For this review, take the finished solid that the model builds, in its own axes (mm). Face numbers are marked on the shaded views. A direction names the side the tool comes from. Give positions to 0.01 mm unless a question says otherwise; leave off trailing zeros. Write each loop counter-clockwise with the first axis right and the second up, starting at its lowest first coordinate (ties: lowest second). Pieces come first, ordered by that corner, then holes.
Q1. For line 1 (Y direction, x = -4.75, z = 0.95); line 2 (X direction, y = 3.25, z = 2); line 3 (X direction, y = 1.25, z = -14.5), list the stretches that pass through material, from the lowest coordinate up.
Q2. We need section C-C (x = 10). Write out the cut boundary in (y, z).
Q3. We need section D-D (y = 9.8). Write out the cut boundary in (x, z), then the cut area to 3 significant figures.
Q4. We need section A-A (x = -4.75). Write out the cut boundary in (y, z), then the cut area to 3 significant figures.
Q5. Insertion check: P1, Ø5.5, axis at x = -4.75, y = 14.7, coming from the +Z side; P2, Ø5, axis at y = 5, z = -21, coming from the +X side; P3, Ø3.5, axis at x = 44, y = 8, coming from the -Z side; P4, Ø3.5, axis at x = 45.65, y = 14.7, coming from the +Z side. Each pin has a flat end and moves straight along its axis. Give the tip position at first contact, or say it passes through.
Q6. Mouldability with a two-part tool opening along Z and no side actions: class the marked faces 5, 6 and 7 as released by +Z, released by -Z, zero draft, split by the parting line, or undercut.
Q7. We need section B-B (y = 4.9). Write out the cut boundary in (x, z).
Q8. Machinability: for the marked faces 1, 2, 3 and 4, which of the approach directions +Z, -Z, +X, -X, +Y, -Y give a long, thin tool a straight path to every point of the face, cutting with its end or side? Answer none if there is none.
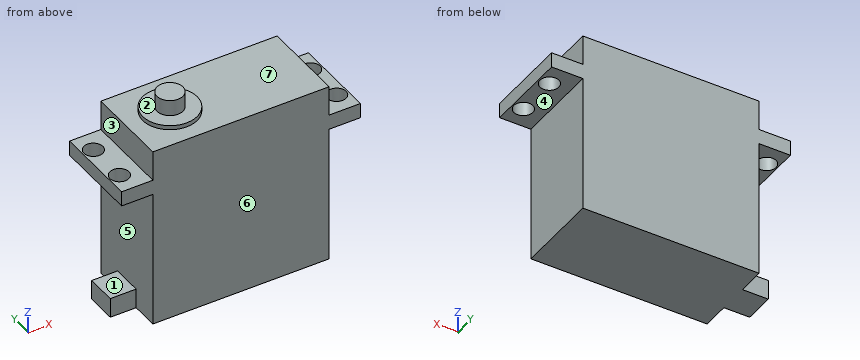
Autodesk Inventor part; units mm, degrees
ref_plane "YZ Plane" through (0, 0, 0) normal (1, 0, 0) x (0, 1, 0)
ref_plane "XZ Plane" through (0, 0, 0) normal (0, 1, 0) x (-1, 0, 0)
ref_plane "XY Plane" through (0, 0, 0) normal (0, 0, 1) x (1, 0, 0)
sketch "Boceto1" plane through (0, 0, 0) normal (0, 1, 0) x (-1, 0, 0)
  line L0 (0, 0) -> (-40.9, 0)
  line L1 (-40.9, 0) -> (-40.9, -32)
  line L2 (-40.9, -32) -> (0, -32)
  line L3 (0, -32) -> (0, 0)
  dimension "d0" = 40.9
  dimension "d1" = 32
extrude "Extrusión1" add sketch "Boceto1" along normal blind 19.6
sketch "Boceto2" plane through (0, 0, 0) normal (0, 0, 1) x (1, 0, 0)
  line L0 (20.45, 29.4794) -> (20.45, -8.3561)
  line L1 (0, 0) -> (0, 19.6)
  line L2 (0, 0) -> (0, 19.6)
  line L3 (20.45, 19.6) -> (-7.25, 19.6)
  line L4 (-7.25, 19.6) -> (-7.25, 0)
  line L5 (-7.25, 0) -> (20.45, 0)
  line L6 (0, 19.6) -> (40.9, 19.6)
  line L7 (0, 0) -> (40.9, 0)
  line L8 (-4.75, 38.1258) -> (-4.75, -18.5214)
  line L9 (50.1495, 9.8) -> (-24.2217, 9.8)
  circle A0 centre (-4.75, 14.7) radius 2.2
  circle A1 centre (-4.75, 4.9) radius 2.2
  line L10 (20.45, 0) -> (0, 0)
  line L11 (40.9, 19.6) -> (0, 19.6)
  line L12 (20.45, 0) -> (40.9, 0)
  line L13 (20.45, 19.6) -> (48.15, 19.6)
  line L14 (48.15, 19.6) -> (48.15, 0)
  line L15 (48.15, 0) -> (20.45, 0)
  circle A2 centre (45.65, 14.7) radius 2.2
  circle A3 centre (45.65, 4.9) radius 2.2
  dimension "d9" = 19.6
  dimension "d10" = 4.4
  dimension "d11" = 9.8
  dimension "d13" = 55.4
  dimension "d14" = 40.9
  dimension "d16" = 25.2
extrude "Extrusión2" add sketch "Boceto2" along normal blind 3.5 contours L6 L13 L14 L9 L0 | L0 L9 L1 L3 | L9 L14 L15 L7 L0 | L0 L5 L1 L9 | L1 L9 L8 A0 L3 | L1 L5 L8 A1 L9 | L8 A0 L9 L4 L3 | L8 A1 L5 L4 L9
sketch "Boceto3" plane through (0, 0, 3.5) normal (0, 0, 1) x (1, 0, 0)
  line L0 (0, 0) -> (40.9, 0)
  line L1 (40.9, 0) -> (40.9, 19.6)
  line L2 (40.9, 19.6) -> (0, 19.6)
  line L3 (0, 19.6) -> (0, 0)
extrude "Extrusión3" add sketch "Boceto3" along normal blind 7
sketch "Boceto4" plane through (0, 0, 10.5) normal (0, 0, 1) x (1, 0, 0)
  circle A0 centre (10, 9.8) radius 6.3
  line L0 (0, 0) -> (40.9, 0)
  line L1 (0, 19.6) -> (0, 0)
  dimension "d21" = 12.6
  dimension "d22" = 9.8
  dimension "d23" = 10
extrude "Extrusión4" add sketch "Boceto4" along normal blind 1
sketch "Boceto5" plane through (10, 9.8, 11.5) normal (0, 0, 1) x (1, 0, 0)
  circle A0 centre (0, 0) radius 3
  circle A1 centre (0, 0) radius 6.3
  point P0 (-10, -9.8)
  dimension "d26" = 6
extrude "Extrusión5" add sketch "Boceto5" along normal blind 3.7 contours A0
sketch "Boceto6" plane through (0, 0, -32) normal (-1, 0, 0) x (0, 0, 1)
  line L0 (0, 0) -> (0, 19.6)
  line L1 (0, 13.3) -> (4.6057, 13.3)
  line L2 (4.6057, 13.3) -> (4.6057, 6.3)
  line L3 (4.6057, 6.3) -> (0, 6.3)
  line L4 (0, 6.3) -> (0, 13.3)
  line L5 (0, 19.6) -> (32, 19.6)
  line L6 (0, 0) -> (32, 0)
  dimension "d29" = 7
  dimension "d30" = 6.3
  dimension "d31" = 6.3
extrude "Extrusión6" add sketch "Boceto6" along normal blind 6
properties part number "savox"
Computed:
1. line 1: y = 0 to 2.7, 7.1 to 12.5, 16.9 to 19.6
1. line 2: x = -7.25 to -6.21, -3.29 to 44.19, 47.11 to 48.15
1. line 3: x = 0 to 40.9
2. outline: (0, -32) - (19.6, -32) - (19.6, 10.5) - (16.1, 10.5) - (16.1, 11.5) - (12.8, 11.5) - (12.8, 15.2) - (6.8, 15.2) - (6.8, 11.5) - (3.5, 11.5) - (3.5, 10.5) - (0, 10.5) - close
3. outline: (-7.25, 0) - (0, 0) - (0, -27.39) - (-6, -27.39) - (-6, -32) - (40.9, -32) - (40.9, 0) - (48.15, 0) - (48.15, 3.5) - (40.9, 3.5) - (40.9, 10.5) - (16.3, 10.5) - (16.3, 11.5) - (13, 11.5) - (13, 15.2) - (7, 15.2) - (7, 11.5) - (3.7, 11.5) - (3.7, 10.5) - (0, 10.5) - (0, 3.5) - (-7.25, 3.5) - close
3. area: 1,850 mm2
4. outline: (0, 0) - (2.7, 0) - (2.7, 3.5) - (0, 3.5) - close; (6.3, -32) - (13.3, -32) - (13.3, -27.39) - (6.3, -27.39) - close; (7.1, 0) - (12.5, 0) - (12.5, 3.5) - (7.1, 3.5) - close; (16.9, 0) - (19.6, 0) - (19.6, 3.5) - (16.9, 3.5) - close
4. area: 70.0 mm2
5. P1: stops at z = 3.5
5. P2: stops at x = 40.9
5. P3: stops at z = 0
5. P4: passes through
6. face 5: undercut
6. face 6: zero draft
6. face 7: released by +Z
7. outline: (-7.25, 0) - (-6.95, 0) - (-6.95, 3.5) - (-7.25, 3.5) - close; (-2.55, 0) - (0, 0) - (0, -32) - (40.9, -32) - (40.9, 0) - (43.45, 0) - (43.45, 3.5) - (40.9, 3.5) - (40.9, 10.5) - (13.96, 10.5) - (13.96, 11.5) - (6.04, 11.5) - (6.04, 10.5) - (0, 10.5) - (0, 3.5) - (-2.55, 3.5) - close; (47.85, 0) - (48.15, 0) - (48.15, 3.5) - (47.85, 3.5) - close
8. face 1: -X, +Y, -Y
8. face 2: +Z
8. face 3: +Z, -X, +Y, -Y
8. face 4: -Z, +X, +Y, -Y
